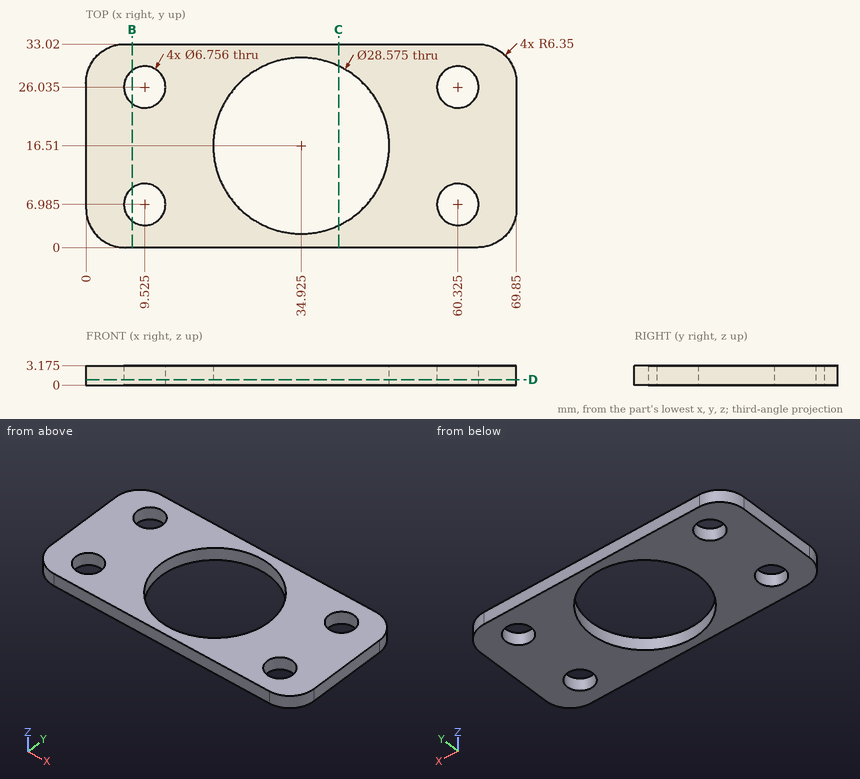
Could you check a few things on this drawing? It's one solid part, dimensions in mm from its lowest x, y, z. Round coordinates to 2 decimals unless told otherwise and drop trailing zeros. Loops run counter-clockwise (first coordinate to the right, second up) from the corner with the lowest first, then second, coordinate; pieces in that order, holes last.
Q1. I want a section at B-B (x = 7.5). Write out the boundary of the cut face in (y, z) (1 decimal).
Q2. I want a section at D-D (z = 0.9). Give the number of separate pieces and of enclosed holes in the cut face, and give its area (3 significant figures).
Q3. For P1, Ø1, axis at y = 29.5, z = 1.5, coming from the +X side, with a flat end and sliding along its axis, tell me the tip position at first contact or that it passes through.
Q4. Please list where these lines run through material, in increasing order: L1, parallel to X at y = 5.5, z = 1.65 (1 decimal); L2, parallel to X at y = 24, z = 1.3; L3, parallel to Y at x = 57.5, z = 2.3 (1 decimal).
Q5. I want a section at C-C (x = 41). Write out the boundary of the cut face in (y, z) (1 decimal).
Answer below:
1. outline: (0, 0) - (4.3, 0) - (4.3, 3.2) - (0, 3.2) - close; (9.7, 0) - (23.3, 0) - (23.3, 3.2) - (9.7, 3.2) - close; (28.7, 0) - (33, 0) - (33, 3.2) - (28.7, 3.2) - close
2. separate pieces: 1
2. enclosed holes: 5
2. area: 1,490 mm2
3. P1: stops at x = 69.41
4. L1: x = 0.1 to 6.5, 12.6 to 25.8, 44 to 57.3, 63.4 to 69.8
4. L2: x = 0 to 6.83, 12.22 to 22.76, 47.09 to 57.63, 63.02 to 69.85
4. L3: y = 0 to 5.1, 8.8 to 24.2, 27.9 to 33
5. outline: (0, 0) - (3.6, 0) - (3.6, 3.2) - (0, 3.2) - close; (29.4, 0) - (33, 0) - (33, 3.2) - (29.4, 3.2) - close
